Source: CAD feature listing. Evaluate the final solid. Frame: model axes, mm. Round coordinates to 2 decimals unless told otherwise and drop trailing zeros. Loops run counter-clockwise (first coordinate to the right, second up) from the corner with the lowest first, then second, coordinate; pieces in that order, holes last.
(1) Section B-B, the plane x = 433.5. Return the cut outline in (y, z).
(2) First-contact query: pin 1 Ø2 at (x, y) = (314.5, -4) entering from +Z; pin 2 Ø2 at (x, y) = (287.5, -16.5) entering from -Z. Flat tips, straight axial feed; report the tip coordinate or a pass-through.
(3) Section A-A, the plane z = -3.3. Return the cut outline in (x, y), plus the area to 3 significant figures.
(4) Section C-C, the plane y = -4.5. Return the cut outline in (x, z), plus the area to 3 significant figures.
(5) Material intervals for probe 1 along Y at (x, z) = (108, -3.55); probe 2 along Z at (x, y) = (428, 13); probe 3 along Y at (x, z) = (146, -5.05), sorted ascending.
```python
from build123d import *

# Parameters (mm, degrees)
EXTRUDE_3_DEPTH = 550


with BuildPart() as part:
    # Эскиз1 → Вытянуть-Тонкостенный3 (new body)
    with BuildSketch(Plane(origin=(0, 0, 0), x_dir=(0, 0, -1), z_dir=(1, 0, 0))):
        with BuildLine():
            Line((6, -18), (6, -20))
            ThreePointArc((6, -20), (5.707106781, -20.707106781), (5, -21))
            Line((5, -21), (1, -21))
            ThreePointArc((1, -21), (0.292893219, -20.707106781), (0, -20))
            Line((0, -20), (0, 20))
            ThreePointArc((0, 20), (0.292893219, 20.707106781), (1, 21))
            Line((1, 21), (5, 21))
            ThreePointArc((5, 21), (5.707106781, 20.707106781), (6, 20))
            Line((6, 20), (6, 18))
            Line((6, 18), (4.8, 18))
            Line((4.8, 18), (4.8, 19.8))
            Line((4.8, 19.8), (1.2, 19.8))
            Line((1.2, 19.8), (1.2, -19.8))
            Line((1.2, -19.8), (4.8, -19.8))
            Line((4.8, -19.8), (4.8, -18))
            Line((4.8, -18), (6, -18))
        make_face()
    extrude(amount=EXTRUDE_3_DEPTH)


solid = part.part
```
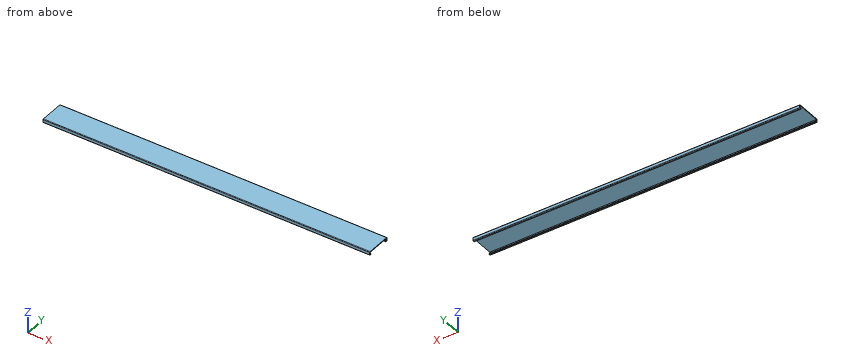
Output values:
1. outline: (-21, -5) arc R1 ccw to (-20, -6) - (-18, -6) - (-18, -4.8) - (-19.8, -4.8) - (-19.8, -1.2) - (19.8, -1.2) - (19.8, -4.8) - (18, -4.8) - (18, -6) - (20, -6) arc R1 ccw to (21, -5) - (21, -1) arc R1 ccw to (20, 0) - (-20, 0) arc R1 ccw to (-21, -1) - close
2. pin 1: stops at z = 0
2. pin 2: stops at z = -1.2
3. outline: (0, -21) - (550, -21) - (550, -19.8) - (0, -19.8) - close; (0, 19.8) - (550, 19.8) - (550, 21) - (0, 21) - close
3. area: 1,320 mm2
4. outline: (0, -1.2) - (550, -1.2) - (550, 0) - (0, 0) - close
4. area: 660 mm2
5. probe 1: y = -21 to -19.8, 19.8 to 21
5. probe 2: z = -1.2 to 0
5. probe 3: y = -21 to -18, 18 to 21
